from build123d import *

# Parameters (mm, degrees)
SKETCH1_R               = 23.5
SKETCH1_R_2             = 21.5
BOSS_EXTRUDE1_DEPTH     = 40
SKETCH3_R               = 23.5
BOSS_EXTRUDE4_DEPTH     = 2
SKETCH4_R               = 7.5
SKETCH4_R_2             = 5.5
BOSS_EXTRUDE5_DEPTH     = 40
SKETCH5_R               = 5.5
CUT_EXTRUDE1_DEPTH      = 41
CUT_EXTRUDE1_DEPTH_BACK = 43


with BuildPart() as part:
    # Sketch1 → Boss-Extrude1 (new body)
    with BuildSketch(Plane.XY):
        Circle(SKETCH1_R)
        Circle(SKETCH1_R_2, mode=Mode.SUBTRACT)
    extrude(amount=BOSS_EXTRUDE1_DEPTH)

    # Sketch3 → Boss-Extrude4 (add)
    with BuildSketch(Plane(origin=(0, 0, 0), x_dir=(-1, 0, 0), z_dir=(0, 0, -1))):
        Circle(SKETCH3_R)
    extrude(amount=BOSS_EXTRUDE4_DEPTH)

    # Sketch4 → Boss-Extrude5 (add)
    with BuildSketch(Plane(origin=(0, 0, -2), x_dir=(-1, 0, 0), z_dir=(0, 0, -1))):
        Circle(SKETCH4_R)
        Circle(SKETCH4_R_2, mode=Mode.SUBTRACT)
    extrude(amount=BOSS_EXTRUDE5_DEPTH)

    # Sketch5 → Cut-Extrude1 (cut, two sides)
    with BuildSketch(Plane(origin=(0, 0, -2), x_dir=(-1, 0, 0), z_dir=(0, 0, -1))) as cut_extrude1_sk:
        Circle(SKETCH5_R)
    extrude(amount=CUT_EXTRUDE1_DEPTH, mode=Mode.SUBTRACT)
    extrude(cut_extrude1_sk.sketch, amount=-CUT_EXTRUDE1_DEPTH_BACK, mode=Mode.SUBTRACT)


solid = part.part
Read the model definition and answer for the solid it produces. Units are mm, in the model's axes. Coordinates: 2 decimals unless noted, no trailing zeros. Write each loop counter-clockwise with the first axis right and the second up, starting at its lowest first coordinate (ties: lowest second). Pieces come first, ordered by that corner, then holes. Notation, with made-up numbers: (18, 40) -> (70, 40) arc R26 ccw to (70, 70) -> close; hole circle Ø11 at (32, 88.25). An arc over 180 degrees is marked (long way). Return JSON: item names as keys, results as strings.
(1) Consider line 1 along Y through (x, z) = (0, 17); line 2 along Y through (x, z) = (0, -0.9); line 3 along Z through (x, y) = (-18.5, 3.5). Determine where each line is inside the solid, lowest interval first. Write a range as from..to.
Answers below:
{"line 1": "-23.5..-21.5, 21.5..23.5", "line 2": "-23.5..-5.5, 5.5..23.5", "line 3": "-2..0"}
(2) The part is cut by section D-D on y = 11. Give the vertices of the cut face in (x, z).
Answers below:
{"outline": "(-20.77, -2) -> (20.77, -2) -> (20.77, 40) -> (18.47, 40) -> (18.47, 0) -> (-18.47, 0) -> (-18.47, 40) -> (-20.77, 40) -> close"}
(3) For a pull along X with two mould halves and no side action, classify faces 1 (the flat face through (-4, -4, 0)), 2 (the cylindrical face through (7.493, 0.33, -21.72)), 3 (the flat face through (6, 6, -2)), 4 (the cylindrical face through (-2.799, 21.317, 19.72)) as pulls with the +X half, pulls with the -X half, needs draft (parallel to the pull), parting line crosses it, or undercut.
Answers below:
{"face 1": "undercut", "face 2": "parting line crosses it", "face 3": "needs draft", "face 4": "undercut"}
(4) The part is cut by section A-A on x = 0. Give the vertices of the cut face in (y, z).
Answers below:
{"outline": "(-23.5, -2) -> (-7.5, -2) -> (-7.5, -42) -> (-5.5, -42) -> (-5.5, 0) -> (-21.5, 0) -> (-21.5, 40) -> (-23.5, 40) -> close; (5.5, -42) -> (7.5, -42) -> (7.5, -2) -> (23.5, -2) -> (23.5, 40) -> (21.5, 40) -> (21.5, 0) -> (5.5, 0) -> close"}
(5) Each of these flat-tipped pins is pushed along its axis until it touches: P1, Ø5, axis at x = 2, z = 29.5, coming from the +Y side; P2, Ø12.5, axis at x = 0, y = 0, coming from the -Z side; P3, Ø1, axis at y = 16.5, z = 4.5, coming from the +X side; P4, Ø3, axis at x = -16.5, y = -8, coming from the -Z side. Where does it stop, or does it pass through?
Answers below:
{"P1": "y = 23.5", "P2": "z = -42", "P3": "x = 17.21", "P4": "z = -2"}
(6) The part is cut by section C-C on z = -34. Give the vertices of the cut face in (x, y).
Answers below:
{"outline": "circle Ø15 at (0, 0); hole circle Ø11 at (0, 0)"}
